Job drawing, mm, ordinate dimensions from the low corner. One solid piece. A direction names the side the tool comes from. Coordinates: 2 decimals unless noted, no trailing zeros. Write each loop counter-clockwise with the first axis right and the second up, starting at its lowest first coordinate (ties: lowest second). Pieces come first, ordered by that corner, then holes.
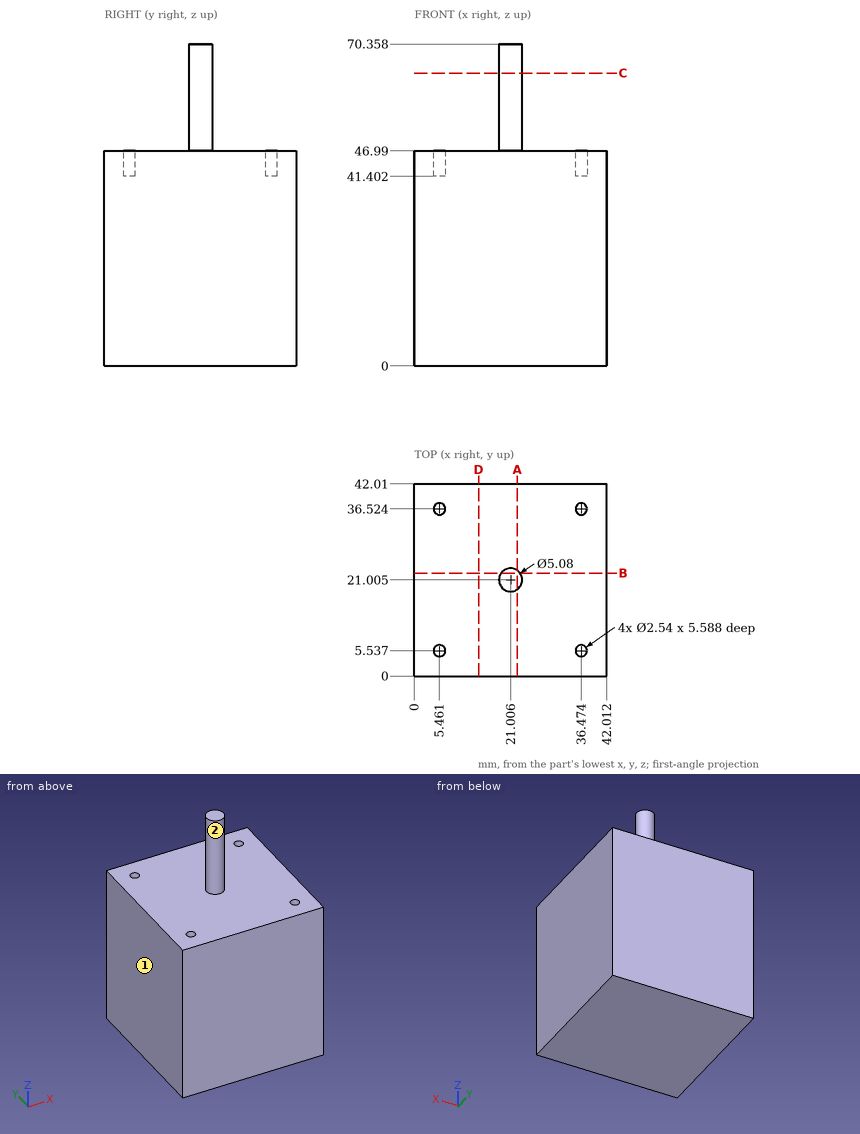
1. 3-axis set-ups, long thin cutter, end or side, ignore diameter. For the marked faces 1 and 2: which of +Z, -Z, +X, -X, +Y, -Y reach the whole face in a straight line?
Computed values:
face 1: +Z, -Z, -X, +Y, -Y
face 2: +Z
2. Probe line 1 along Z through (x, y) = (16, 6); line 2 along Z through (x, y) = (36, 37.5). List the from-to ranges inside material, lowest first.
Computed values:
line 1: z = 0 to 46.99
line 2: z = 0 to 41.4
3. Flat gauge pins, fed straight in: pin 1 (3 mm diameter, centred on x = 36.47, y = 36.52, fed in from +Z); pin 2 (6 mm diameter, centred on x = 17, z = 59.5, fed in from -Y); pin 3 (0.8 mm diameter, centred on x = 37, y = 37, fed in from +Z). Where does each tip first touch, or does it go through?
Computed values:
pin 1: stops at z = 46.99
pin 2: stops at y = 18.67
pin 3: stops at z = 41.4
4. Saw through at C-C on z = 64. List the corners of the cut face in (x, y) (1 decimal).
Computed values:
outline: circle Ø5.1 at (21, 21)
5. Saw through at D-D on x = 14. List the corners of the cut face in (y, z).
Computed values:
outline: (0, 0) - (42.01, 0) - (42.01, 46.99) - (0, 46.99) - close
6. Saw through at A-A on x = 22.5. List the corners of the cut face in (y, z).
Computed values:
outline: (0, 0) - (42.01, 0) - (42.01, 46.99) - (23.06, 46.99) - (23.06, 70.36) - (18.95, 70.36) - (18.95, 46.99) - (0, 46.99) - close
